Read the model definition and answer for the solid it produces. Units are mm, in the model's axes. A direction names the side the tool comes from. Give positions to 0.01 mm unless a question says otherwise; leave off trailing zeros. Loops run counter-clockwise (first coordinate to the right, second up) from the corner with the lowest first, then second, coordinate; pieces in that order, holes last. Notation, with made-up numbers: (-13, -24.5) - (-1, -24.5) arc R26 ccw to (-1, 2.5) - close; hole circle Ø4 at (44, -16.75). An arc over 180 degrees is marked (long way). Write item = value, one per line. Start each with the question number.
from build123d import *

# Parameters (mm, degrees)
BOSS_EXTRUDE1_DEPTH  = 3
M8_CLEARANCE_HOLE1_D = 9
M3_CLEARANCE_HOLE1_D = 3.4
FILLET1_R            = 1
FILLET2_R            = 7.5
SKETCH6_W            = 80
SKETCH6_H            = 9
CUT_EXTRUDE1_DEPTH   = 112.843640856
FILLET3_R            = 1


with BuildPart() as part:
    # Sketch1 → Boss-Extrude1 (new body)
    with BuildSketch(Plane(origin=(0, 0, 0), x_dir=(1, 0, 0), z_dir=(0, 1, 0))):
        Polygon((0, 0), (0, 20), (110, 20), (110, 5), (10, 5), (10, 0), align=None)
    extrude(amount=BOSS_EXTRUDE1_DEPTH)

    # M8 Clearance Hole1 (through all)
    with Locations(Plane(origin=(100, 3, -12.5), x_dir=(0, 0, 1), z_dir=(0, 1, 0))):
        with Locations((0, 0)):
            Hole(M8_CLEARANCE_HOLE1_D / 2)

    # M3 Clearance Hole1 (through all)
    with Locations(Plane(origin=(5, 3, -15), x_dir=(0, 0, 1), z_dir=(0, 1, 0))):
        with Locations((0, 0), (10, 0)):
            Hole(M3_CLEARANCE_HOLE1_D / 2)

    # Fillet1
    fillet1_edges = [part.edges().sort_by_distance(p)[0] for p in [
        (0, 1.5, 0),
        (0, 1.5, -20),
        (10, 1.5, -5),
        (10, 1.5, 0),
    ]]
    fillet(fillet1_edges, radius=FILLET1_R)

    # Fillet2
    fillet2_edges = [part.edges().sort_by_distance(p)[0] for p in [
        (110, 1.5, -20),
        (110, 1.5, -5),
    ]]
    fillet(fillet2_edges, radius=FILLET2_R - 0.0001)  # a hair under: the kernel refuses the full size

    # Sketch6 → Cut-Extrude1 (cut, through all)
    with BuildSketch(Plane(origin=(0, 3, 0), x_dir=(1, 0, 0), z_dir=(0, 1, 0))):
        with Locations((50, 12.5)):
            Rectangle(SKETCH6_W, SKETCH6_H)
    extrude(amount=-CUT_EXTRUDE1_DEPTH, mode=Mode.SUBTRACT)

    # Fillet3
    fillet3_edges = [part.edges().sort_by_distance(p)[0] for p in [
        (10, 1.5, -8),
        (10, 1.5, -17),
        (90, 1.5, -17),
        (90, 1.5, -8),
    ]]
    fillet(fillet3_edges, radius=FILLET3_R)


solid = part.part
1. For a pull along Z with two mould halves and no side action, classify faces 1 (the flat face through (5, 1, 0)), 2 (the flat face through (10, 2, -12)), 3 (the cylindrical face through (107.745, 1.521, -17.861)) as released by +Z, released by -Z, zero draft, split by the parting line, or undercut.
2. Consider line 1 along X through (y, z) = (2.55, -12.75); line 2 along Z through (x, y) = (37, 1.15); line 3 along X through (y, z) = (2.1, -15). Determine where each line is inside the solid, lowest interval first. Write a range as [from, to].
3. A cutting plane is placed at D-D on z = -15. Give the vertices of the cut face in (x, y), and give its area (3 significant figures).
4. A cutting plane is placed at B-B on x = 100. Give the vertices of the cut face in (y, z), and give its area (3 significant figures).
5. A tool of negligible diameter and unlimited length cuts with its end or side. For faces 4 (the flat face through (10, 1, -3)), 5 (the flat face through (0, 1, -10)), 6 (the flat face through (49, 2, -8)), from which of +Z, -Z, +X, -X, +Y, -Y can it reach the whole face along a straight path? Write none if from no direction.
6. A cutting plane is placed at A-A on y = 2.3. Give the number of separate pieces and of enclosed holes in the cut face, and give its area (3 significant figures).
7. A cutting plane is placed at C-C on x = 5. Give the vertices of the cut face in (y, z).
Reply:
q1.face_1 = released by +Z
q1.face_2 = undercut
q1.face_3 = released by -Z
q2.line_1 = [0, 10], [90, 95.51], [104.49, 110]
q2.line_2 = [-20, -17], [-8, -5]
q2.line_3 = [0, 3.3], [6.7, 10], [90, 96.26], [103.74, 109.57]
q3.outline = (0, 0) - (3.3, 0) - (3.3, 3) - (0, 3) - close; (6.7, 0) - (10, 0) - (10, 3) - (6.7, 3) - close; (90, 0) - (96.26, 0) - (96.26, 3) - (90, 3) - close; (103.74, 0) - (109.57, 0) - (109.57, 3) - (103.74, 3) - close
q3.area = 56.1 mm^2
q4.outline = (0, -20) - (3, -20) - (3, -17) - (0, -17) - close; (0, -8) - (3, -8) - (3, -5) - (0, -5) - close
q4.area = 18.0 mm^2
q5.face_4 = +Z, +X, +Y, -Y
q5.face_5 = +Z, -Z, -X, +Y, -Y
q5.face_6 = +Y, -Y
q6.separate_pieces = 1
q6.enclosed_holes = 4
q6.area = 875 mm^2
q7.outline = (0, -20) - (3, -20) - (3, -16.7) - (0, -16.7) - close; (0, -13.3) - (3, -13.3) - (3, -6.7) - (0, -6.7) - close; (0, -3.3) - (3, -3.3) - (3, 0) - (0, 0) - close
